from build123d import *

# Parameters (mm, degrees)
BOSS_EXTRUDE1_DEPTH = 20
SKETCH1_3_R         = 20
SKETCH1_3_R_2       = 15
SKETCH1_3_R_3       = 27.5
SKETCH1_3_R_4       = 6
BOSS_EXTRUDE2_DEPTH = 30


with BuildPart() as part:
    # Sketch1 → Boss-Extrude1 (new body)
    with BuildSketch(Plane.XY):
        with BuildLine():
            Line((72.289579528, -103.395415906), (84.84696693, -2.469393386))
            ThreePointArc((84.84696693, -2.469393386), (57.710349886, -18.624204714), (48.75, 11.659223816))
            ThreePointArc((48.75, 11.659223816), (32.5, 3.318447633), (16.25, 11.659223816))
            ThreePointArc((16.25, 11.659223816), (19.039432765, 6.123724357), (20, 0))
            ThreePointArc((20, 0), (-4.490678851, -19.489325372), (-17.983380346, 8.752030126))
            ThreePointArc((-17.983380346, 8.752030126), (-20.994881076, -70.178879235), (35.195495857, -125.692833602))
            ThreePointArc((35.195495857, -125.692833602), (29.401504302, -77.351888998), (72.5, -100))
            ThreePointArc((72.5, -100), (72.447344471, -101.700964869), (72.289579528, -103.395415906))
        make_face()
    extrude(amount=BOSS_EXTRUDE1_DEPTH)

    # Sketch1_3 → Boss-Extrude2 (add)
    # profile 1 of 3: a face of its own
    with BuildSketch(Plane.XY):
        with Locations(Location((0, 0, 0), (0, 0, 154.04905234))):
            Circle(SKETCH1_3_R)
        Circle(SKETCH1_3_R_2, mode=Mode.SUBTRACT)
    # profile 2 of 3: a face of its own
    with BuildSketch(Plane.XY):
        with Locations(Location((65, 0, 0), (0, 0, 144.340912304))):
            Circle(SKETCH1_3_R)
        with Locations((65, 0)):
            Circle(SKETCH1_3_R_2, mode=Mode.SUBTRACT)
    # profile 3 of 3: a face of its own
    with BuildSketch(Plane.XY):
        with Locations(Location((45, -100, 0), (0, 0, 249.112914296))):
            Circle(SKETCH1_3_R_3)
        with Locations((26, -100)):
            Circle(SKETCH1_3_R_4, mode=Mode.SUBTRACT)
        with Locations((45, -119)):
            Circle(SKETCH1_3_R_4, mode=Mode.SUBTRACT)
        with Locations((64, -100)):
            Circle(SKETCH1_3_R_4, mode=Mode.SUBTRACT)
        with Locations((45, -81)):
            Circle(SKETCH1_3_R_4, mode=Mode.SUBTRACT)
    extrude(amount=BOSS_EXTRUDE2_DEPTH)


solid = part.part
Geometry check sheet. Reference: the model listing, model coordinates, mm. A direction names the side the tool comes from. Give positions to 0.01 mm unless a question says otherwise; leave off trailing zeros. Loops run counter-clockwise (first coordinate to the right, second up) from the corner with the lowest first, then second, coordinate; pieces in that order, holes last. Notation, with made-up numbers: (74.25, 24) -> (102.25, 24) arc R5 cw to (102.25, 32) -> close; hole circle Ø2 at (51, 31). An arc over 180 degrees is marked (long way). Answer in a Markdown table with one row per item. Add a question column.
1) Cross-section at C-C on y = 0. Record the boundary of the cut face in (x, z).
2) Material ranges on probe 1 along Y at (x, z) = (40.5, 1.25); probe 2 along Z at (x, y) = (-22, -57); probe 3 along X at (y, z) = (12, 5), recorded low to high. Write a range as from..to.
3) Cross-section at D-D on x = 76. Record the boundary of the cut face in (y, z).
4) Set-up check for faces 1 (the face through (61.39, -122.08, 18.12)), 2 (the face through (44.22, -113.05, 14.79)): record each of +Z, -Z, +X, -X, +Y, -Y from which the full face is reachable in a straight line by a thin tool's end or side.
5) Gauge pin test, flat ends, axial feed: P1, Ø7, axis at x = 64, y = -100, coming from the +Z side; P2, Ø1, axis at x = 18.5, z = 23.5, coming from the +Y side; P3, Ø2, axis at x = 63, z = 16.5, coming from the -Y side; P4, Ø10, axis at y = -100, z = 12, coming from the +X side. Record the tip position at first contact, or that the pin passes through.
6) Cross-section at B-B on z = 26.75. State how many separate pieces and enclosed holes the cut face has, and give its area (3 significant figures).
7) Draft check along X on faces 3 (the face through (50.015, 0.66, 14.79)), 4 (the face through (40.58, -76.94, 14.79)), 5 (the face through (-21.407, -69.118, 9.86)), 6 (the face through (53.98, -10.44, 30)). Enter one of: pulls with the +X half, pulls with the -X half, needs draft (parallel to the pull), parting line crosses it, or undercut.
8) Cross-section at A-A on x = 64. Record the boundary of the cut face in (y, z).
Outcome:
| question | item | result |
|---|---|---|
| 1 | outline | (-21.73, 0) -> (-15, 0) -> (-15, 30) -> (-20, 30) -> (-20, 20) -> (-21.73, 20) -> close; (15, 0) -> (50, 0) -> (50, 30) -> (45, 30) -> (45, 20) -> (20, 20) -> (20, 30) -> (15, 30) -> close; (80, 0) -> (85, 0) -> (85, 30) -> (80, 30) -> close |
| 2 | probe 1 | y = -127.13..-122.97, -115.03..-84.97, -77.03..4.99 |
| 2 | probe 2 | z = 0..20 |
| 2 | probe 3 | x = -16..-9, 9..16, 49..56, 74..81 |
| 3 | outline | (-73.57, 0) -> (-10.2, 0) -> (-10.2, 30) -> (-16.7, 30) -> (-16.7, 20) -> (-73.57, 20) -> close; (10.2, 0) -> (16.7, 0) -> (16.7, 30) -> (10.2, 30) -> close |
| 4 | face 1 | +Z |
| 4 | face 2 | +Z, -Z |
| 5 | P1 | passes through |
| 5 | P2 | stops at y = 8.72 |
| 5 | P3 | stops at y = -121.62 |
| 5 | P4 | stops at x = 73.33 |
| 6 | separate pieces | 3 |
| 6 | enclosed holes | 6 |
| 6 | area | 3,020 mm^2 |
| 7 | face 3 | undercut |
| 7 | face 4 | undercut |
| 7 | face 5 | pulls with the -X half |
| 7 | face 6 | needs draft |
| 8 | outline | (-119.88, 0) -> (-106, 0) -> (-106, 30) -> (-119.88, 30) -> close; (-94, 0) -> (-14.97, 0) -> (-14.97, 30) -> (-19.97, 30) -> (-19.97, 20) -> (-80.12, 20) -> (-80.12, 30) -> (-94, 30) -> close; (14.97, 0) -> (19.97, 0) -> (19.97, 30) -> (14.97, 30) -> close |
